```python
from build123d import *

# Parameters (mm, degrees)
SKETCH1_R           = 7.75
BOSS_EXTRUDE1_DEPTH = 4
FILLET1_R           = 0.05


with BuildPart() as part:
    # Sketch1 → Boss-Extrude1 (new body)
    with BuildSketch(Plane.XY):
        Circle(SKETCH1_R)
    extrude(amount=BOSS_EXTRUDE1_DEPTH)

    # Sketch2 → Cut-Revolve1 (revolve, cut)
    with BuildSketch(Plane(origin=(0, 0, 0), x_dir=(0, 0, -1), z_dir=(1, 0, 0)), mode=Mode.PRIVATE) as cut_revolve1_sk:
        with BuildLine():
            Line((-0.4, 0.91), (-2.1, 0.91))
            ThreePointArc((-2.1, 0.91), (-2.743467171, 0.643467171), (-3.01, 0))
            Line((-3.01, 0), (0.05, 0))
            Line((0.05, 0), (0.05, 1.08))
            Line((0.05, 1.08), (-0.4, 1.08))
            Line((-0.4, 1.08), (-0.4, 0.91))
        make_face()
    revolve(cut_revolve1_sk.sketch.rotate(Axis((0, 0, 3.01), (0, 0, -1)), 180), axis=Axis((0, 0, 3.01), (0, 0, -1)), mode=Mode.SUBTRACT)

    # Fillet1
    fillet1_edges = [part.edges().sort_by_distance(p)[0] for p in [
        (0, 0.91, 0.4),
    ]]
    fillet(fillet1_edges, radius=FILLET1_R)


solid = part.part
```
Geometry: final body of the model. Coordinates: model frame, mm. A direction names the side the tool comes from. Coordinates: 2 decimals unless noted, no trailing zeros. Order: outer loops, then holes, each group sorted by start corner. A loop starts at its lowest first (then second) coordinate and runs counter-clockwise, first axis right, second up. Notation, with made-up numbers: (24.5, 52) - (43.5, 52) arc R21 cw to (43.5, 77) - close; hole circle Ø1 at (77, -32.75). An arc over 180 degrees is marked (long way). Return JSON: item names as keys, results as strings. Group by question number.
1. Material intervals for line 1 along Y through (x, z) = (0.25, 1.7); line 2 along Y through (x, z) = (3.5, 2.8); line 3 along Y through (x, z) = (3.25, 2.2), sorted ascending. Write a range as [from, to].
2. Pull-direction query (X, two-part tool) for faces 1 (the face through (-1.009, 7.684, 1.972)), 2 (the face through (0, -2, 0)), 3 (the face through (-0.32, -1.03, 0.2)); classes: pulls with the +X half, pulls with the -X half, needs draft (parallel to the pull), parting line crosses it, or undercut.
3. Set-up query: faces 4 (the face through (0.807, -0.42, 1.287)), 5 (the face through (0, 0, 4)). Return all of +Z, -Z, +X, -X, +Y, -Y with unobstructed straight access to the full face (end or side cutting, diameter ignored); none if empty.
4. Cut plane C-C (z = 1.6). Output: boundary loops of the cut face in (x, y), plus the area to 3 significant figures.
5. Pin query (flat end, axial travel): pin 1 (6 mm diameter, centred on x = -4, y = -3, fed in from -Z); pin 2 (2 mm diameter, centred on x = 3.5, z = 1.5, fed in from +Y). Return the tip coordinate at first contact, or that it passes through.
6. Cut plane A-A (x = 0). Output: boundary loops of the cut face in (y, z).
7. Cut plane D-D (y = -6). Output: boundary loops of the cut face in (x, z), plus the area to 3 significant figures.
Resolved:
{
 "1": {"line 1": "y = [-7.75, -0.87], [0.87, 7.75]", "line 2": "y = [-6.91, 6.91]", "line 3": "y = [-7.04, 7.04]"},
 "2": {"face 1": "parting line crosses it", "face 2": "needs draft", "face 3": "undercut"},
 "3": {"face 4": "-Z", "face 5": "+Z, +X, -X, +Y, -Y"},
 "4": {"outline": "circle Ø15.5 at (0, 0); hole circle Ø1.82 at (0, 0)", "area": "186 mm²"},
 "5": {"pin 1": "stops at z = 0", "pin 2": "stops at y = 7.34"},
 "6": {"outline": "(-7.75, 0) - (-1.08, 0) - (-1.08, 0.4) - (-0.96, 0.4) arc R0.05 ccw to (-0.91, 0.45) - (-0.91, 2.1) arc R0.91 cw to (0.91, 2.1) - (0.91, 0.45) arc R0.05 ccw to (0.96, 0.4) - (1.08, 0.4) - (1.08, 0) - (7.75, 0) - (7.75, 4) - (-7.75, 4) - close"},
 "7": {"outline": "(-4.91, 0) - (4.91, 0) - (4.91, 4) - (-4.91, 4) - close", "area": "39.2 mm²"}
}
